CAD build for the part. Positions are in the model's coordinates, mm. Face numbers are marked on the shaded views. A direction names the side the tool comes from. Give positions to 0.01 mm unless a question says otherwise; leave off trailing zeros. Loops run counter-clockwise (first coordinate to the right, second up) from the corner with the lowest first, then second, coordinate; pieces in that order, holes last.
Item 1: Saw through at D-D on x = 28. Give the cut face in (y, z).
Item 2: Drop flat-ended pins along their axis: P1, Ø2.5, axis at x = -7, z = 0, coming from the +Y side; P2, Ø1, axis at x = 2, y = 3, coming from the +Z side; P3, Ø4, axis at x = -1.5, z = 0.5, coming from the -Y side. Give the stop position or say it passes through.
Item 3: Which spindle directions (+Z, -Z, +X, -X, +Y, -Y) get a long thin tool onto all of the face, cutting with end or side? Do the marked faces 1, 2 and 3. Say none if no direction does.
Item 4: Saw through at A-A on x = -7. Give the cut face in (y, z), plus the area to 3 significant figures.
Item 5: Saw through at B-B on z = -7. Give the cut face in (x, y), plus the area to 3 significant figures.
Item 6: Saw through at C-C on y = 1.75. Give the cut face in (x, z), plus the area to 3 significant figures.
Item 7: Mould opens along X. For the marked faces 4, 5 and 6 say: released by +X, released by -X, zero draft, split by the parting line, or undercut.
Item 8: Probe probe 1 along Z at (x, y) = (0, -0.3); probe 2 along X at (y, z) = (1.55, 0); probe 3 along X at (y, z) = (1.8, 7). List the from-to ranges inside material, lowest first.
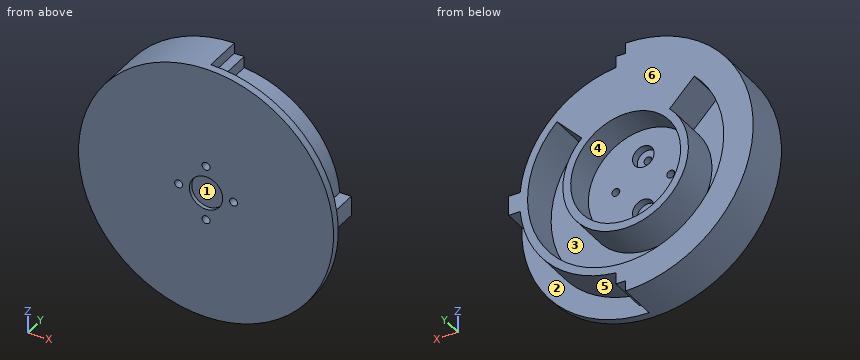
from build123d import *

# Parameters (mm, degrees)
SKETCH1_R               = 27
SKETCH1_R_2             = 14
BOSS_EXTRUDE1_DEPTH     = 10
SKETCH2_R               = 32.5
BOSS_EXTRUDE2_DEPTH     = 2
SKETCH3_W               = 5
SKETCH3_H               = 4.39677325
SKETCH3_W_2             = 4.39677325
SKETCH3_H_2             = 5
BOSS_EXTRUDE3_DEPTH     = 10
BOSS_EXTRUDE4_DEPTH     = 10
BOSS_EXTRUDE5_START     = -2.5
SKETCH6_R               = 14
BOSS_EXTRUDE5_DEPTH     = 2.5
CUT_EXTRUDE1_DEPTH      = 48.502631506
CUT_EXTRUDE1_DEPTH_BACK = 48.502631506
SKETCH4_R               = 1
SKETCH10_R              = 2.75
CUT_EXTRUDE4_DEPTH      = 2
SKETCH11_R              = 4.25
CUT_EXTRUDE5_DEPTH      = 1


with BuildPart() as part:
    # Sketch1 → Boss-Extrude1 (new body)
    with BuildSketch(Plane(origin=(0, 0, 0), x_dir=(1, 0, 0), z_dir=(0, 1, 0))):
        with Locations(Location((0, 0, 0), (0, 0, 270))):
            Circle(SKETCH1_R)
        with Locations(Location((0, 0, 0), (0, 0, 270))):
            Circle(SKETCH1_R_2, mode=Mode.SUBTRACT)
        with BuildLine():
            Line((-17.5, -17.853571071), (-11.2, -11.426285486))
            ThreePointArc((-11.2, -11.426285486), (0, 16), (11.2, -11.426285486))
            Line((11.2, -11.426285486), (17.5, -17.853571071))
            ThreePointArc((17.5, -17.853571071), (0, 25), (-17.5, -17.853571071))
        make_face(mode=Mode.SUBTRACT)
    extrude(amount=BOSS_EXTRUDE1_DEPTH)

    # Sketch2 → Boss-Extrude2 (add)
    with BuildSketch(Plane.XZ):
        with Locations(Location((0, 0, 0), (0, 0, 270))):
            Circle(SKETCH2_R)
    extrude(amount=BOSS_EXTRUDE2_DEPTH)

    # Sketch3 → Boss-Extrude3 (add)
    with BuildSketch(Plane(origin=(0, 0, 0), x_dir=(1, 0, 0), z_dir=(0, 1, 0))):
        with Locations((0, 27.601613375)):
            Rectangle(SKETCH3_W, SKETCH3_H)
        with Locations((27.601613375, 0)):
            Rectangle(SKETCH3_W_2, SKETCH3_H_2)
        with Locations((0, -27.601613375)):
            Rectangle(SKETCH3_W, SKETCH3_H)
        with Locations((-27.601613375, 0)):
            Rectangle(SKETCH3_W_2, SKETCH3_H_2)
    extrude(amount=BOSS_EXTRUDE3_DEPTH)

    # Sketch5 → Boss-Extrude4 (add)
    with BuildSketch(Plane(origin=(0, 0, 0), x_dir=(1, 0, 0), z_dir=(0, 1, 0))):
        with BuildLine():
            Line((0, 29.8), (0, 32.5))
            ThreePointArc((0, 32.5), (-32.5, 0), (0, -32.5))
            Line((0, -32.5), (0, -29.8))
            Line((0, -29.8), (-2.5, -29.8))
            Line((-2.5, -29.8), (-2.5, -26.884010118))
            ThreePointArc((-2.5, -26.884010118), (-19.091883092, -19.091883092), (-26.884010118, -2.5))
            Line((-26.884010118, -2.5), (-29.8, -2.5))
            Line((-29.8, -2.5), (-29.8, 2.5))
            Line((-29.8, 2.5), (-26.884010118, 2.5))
            ThreePointArc((-26.884010118, 2.5), (-19.091883092, 19.091883092), (-2.5, 26.884010118))
            Line((-2.5, 26.884010118), (-2.5, 29.8))
            Line((-2.5, 29.8), (0, 29.8))
        make_face()
    extrude(amount=BOSS_EXTRUDE4_DEPTH)

    # Sketch6 → Boss-Extrude5 (add)
    with BuildSketch(Plane(origin=(0, 2.5, 0), x_dir=(1, 0, 0), z_dir=(0, 1, 0)).offset(BOSS_EXTRUDE5_START)):
        with Locations(Location((0, 0, 0), (0, 0, 270))):
            Circle(SKETCH6_R)
    extrude(amount=BOSS_EXTRUDE5_DEPTH)

    # Sketch4 → Cut-Extrude1 (cut, two sides: drawn at the far end of the back side and taken through both)
    with BuildSketch(Plane.XZ.offset(2).offset(-CUT_EXTRUDE1_DEPTH_BACK)):
        with Locations(Location((0, -7, 0), (0, 0, 270))):
            Circle(SKETCH4_R)
        with Locations(Location((-7, 0, 0), (0, 0, 270))):
            Circle(SKETCH4_R)
        with Locations(Location((0, 7, 0), (0, 0, 270))):
            Circle(SKETCH4_R)
        with Locations(Location((7, 0, 0), (0, 0, 270))):
            Circle(SKETCH4_R)
    extrude(amount=CUT_EXTRUDE1_DEPTH + CUT_EXTRUDE1_DEPTH_BACK, mode=Mode.SUBTRACT)

    # Sketch10 → Cut-Extrude4 (cut)
    with BuildSketch(Plane(origin=(0, 2.5, 0), x_dir=(1, 0, 0), z_dir=(0, 1, 0))):
        with Locations(Location((0, 7, 0), (0, 0, 270))):
            Circle(SKETCH10_R)
        with Locations(Location((0, -7, 0), (0, 0, 270))):
            Circle(SKETCH10_R)
    extrude(amount=-CUT_EXTRUDE4_DEPTH, mode=Mode.SUBTRACT)

    # Sketch11 → Cut-Extrude5 (cut)
    with BuildSketch(Plane.XZ.offset(2)):
        with Locations(Location((0, 0, 0), (0, 0, 270))):
            Circle(SKETCH11_R)
    extrude(amount=-CUT_EXTRUDE5_DEPTH, mode=Mode.SUBTRACT)


solid = part.part
Results below:
1. outline: (-2, -16.5) - (0, -16.5) - (0, -2.5) - (10, -2.5) - (10, 2.5) - (0, 2.5) - (0, 16.5) - (-2, 16.5) - close
2. P1: stops at y = 2.5
2. P2: stops at z = 29.8
2. P3: stops at y = -1
3. face 1: -Y
3. face 2: +X, +Y
3. face 3: +Y
4. outline: (-2, -31.74) - (10, -31.74) - (10, -24) - (0, -24) - (0, -14.39) - (10, -14.39) - (10, -12.12) - (2.5, -12.12) - (2.5, -1) - (-2, -1) - close; (-2, 1) - (2.5, 1) - (2.5, 12.12) - (10, 12.12) - (10, 31.74) - (-2, 31.74) - close
4. area: 475 mm2
5. outline: (-31.74, -2) - (-1, -2) - (-1, 0.5) - (-2.75, 0.5) - (-2.75, 2.5) - (-12.12, 2.5) - (-12.12, 10) - (-14.39, 10) - (-14.39, 0) - (-24, 0) - (-24, 10) - (-31.74, 10) - close; (1, -2) - (31.74, -2) - (31.74, 0) - (26.08, 0) - (26.08, 10) - (24, 10) - (24, 0) - (14.39, 0) - (14.39, 10) - (12.12, 10) - (12.12, 2.5) - (2.75, 2.5) - (2.75, 0.5) - (1, 0.5) - close
5. area: 315 mm2
6. outline: (0, -32.5) - (0, -29.8) - (2.5, -29.8) - (2.5, -26.88) arc R27 ccw to (26.88, -2.5) - (29.8, -2.5) - (29.8, 2.5) - (26.88, 2.5) arc R27 ccw to (2.5, 26.88) - (2.5, 29.8) - (0, 29.8) - (0, 32.5) arc R32.5 ccw to start; hole (-17.5, 17.85) arc R25 ccw (long way) to (17.5, 17.85) - (11.2, 11.43) arc R16 cw (long way) to (-11.2, 11.43) - close; hole circle Ø2 at (-7, 0); hole circle Ø5.5 at (0, -7); hole circle Ø5.5 at (0, 7); hole circle Ø2 at (7, 0)
6. area: 1,910 mm2
7. face 4: undercut
7. face 5: released by +X
7. face 6: zero draft
8. probe 1: z = -32.5 to -8, -6 to 6, 8 to 32.5
8. probe 2: x = -32.5 to -25, -16 to -8, -6 to 6, 8 to 16, 25 to 29.8
8. probe 3: x = -31.74 to -24, -14.39 to -2.75, 2.75 to 14.39, 24 to 26.08
